from build123d import *

# Parameters (mm, degrees)
F0_W      = 90
F0_H      = 55
F1_DEPTH  = 40
F2_R      = 25
F3_DEPTH  = 45
F4_R      = 25
F5_DEPTH  = 5
F6_W      = 60
F6_H      = 40
F7_DEPTH  = 20
F8_W      = 30
F8_H      = 30
F9_DEPTH  = 10
F10_W     = 15
F10_H     = 30
F11_DEPTH = 30
F13_DEPTH = 45.001
F14_R     = 15
F15_DEPTH = 10
F16_R     = 15
F17_DEPTH = 10
F18_R     = 15
F19_DEPTH = 10
F20_R     = 15
F21_DEPTH = 10


with BuildPart() as f1:
    # F0 (on Front) → F1 (new body)
    with BuildSketch(Plane.XZ):
        Rectangle(F0_W, F0_H)
    extrude(amount=F1_DEPTH)

    # F2 (on face) → F3 (join)
    with BuildSketch(Plane.XZ.offset(40)):
        with Locations((-45, -27.5)):
            Circle(F2_R)
        with Locations((45, -27.5)):
            Circle(F2_R)
    extrude(amount=-F3_DEPTH)

    # F4 (on face) → F5 (join)
    with BuildSketch(Plane.XZ.offset(40)):
        with Locations((-45, -27.5)):
            Circle(F4_R)
        with Locations((45, -27.5)):
            Circle(F4_R)
    extrude(amount=F5_DEPTH)

    # F6 (on face) → F7 (cut)
    with BuildSketch(Plane.XY.offset(27.5)):
        with Locations((15, -20)):
            Rectangle(F6_W, F6_H)
    extrude(amount=-F7_DEPTH, mode=Mode.SUBTRACT)

    # F8 (on face) → F9 (cut)
    with BuildSketch(Plane.XY.offset(7.5)):
        with Locations((0, -20)):
            Rectangle(F8_W, F8_H)
    extrude(amount=-F9_DEPTH, mode=Mode.SUBTRACT)

    # F10 (on face) → F11 (cut)
    with BuildSketch(Plane.XY.offset(27.5)):
        with Locations((-22.5, -20)):
            Rectangle(F10_W, F10_H)
    extrude(amount=-F11_DEPTH, mode=Mode.SUBTRACT)

    # F12 (on face) → F13 (cut, through all)
    with BuildSketch(Plane.XZ.offset(40)):
        Polygon((-15, 27.5), (-30, 27.5), (-15, 12.5), align=None)
        Polygon((-45, 22.5), (-40, 27.5), (-45, 27.5), align=None)
    extrude(amount=-F13_DEPTH, mode=Mode.SUBTRACT)

    # F14 (on face) → F15 (cut)
    with BuildSketch(Plane.XZ.offset(45)):
        with Locations((-45, -27.5)):
            Circle(F14_R)
    extrude(amount=-F15_DEPTH, mode=Mode.SUBTRACT)

    # F16 (on face) → F17 (cut)
    with BuildSketch(Plane.XZ.offset(45)):
        with Locations((45, -27.5)):
            Circle(F16_R)
    extrude(amount=-F17_DEPTH, mode=Mode.SUBTRACT)

    # F18 (on face) → F19 (cut)
    with BuildSketch(Plane(origin=(0, 5, 0), x_dir=(-1, 0, 0), z_dir=(0, 1, 0))):
        with Locations((-45, -27.5)):
            Circle(F18_R)
    extrude(amount=-F19_DEPTH, mode=Mode.SUBTRACT)

    # F20 (on face) → F21 (cut)
    with BuildSketch(Plane(origin=(0, 5, 0), x_dir=(-1, 0, 0), z_dir=(0, 1, 0))):
        with Locations((45, -27.5)):
            Circle(F20_R)
    extrude(amount=-F21_DEPTH, mode=Mode.SUBTRACT)


solid = f1.part
Design review of the part built by this model. Coordinates are the model's own, in mm. A direction names the side the tool comes from. Round coordinates to 2 decimals unless told otherwise and drop trailing zeros. Loops run counter-clockwise (first coordinate to the right, second up) from the corner with the lowest first, then second, coordinate; pieces in that order, holes last. Notation, with made-up numbers: (11, 67) - (49, 67) arc R11 ccw to (49, 81) - close; hole circle Ø1 at (-24.5, 11). An arc over 180 degrees is marked (long way). One line per question, with ' | ' between items.
1. For faces 5 (the face through (-1, 0, 0)), 6 (the face through (45, -35, -27)), 7 (the face through (-15, -38, 10)), 8 (the face through (59.985, 0.07, -26.84)), 9 (the face through (15, -20, 3)), list the 3-axis set-ups (+Z, -Z, +X, -X, +Y, -Y) from which the entire face can be reached by the end or side of a thin tool; tool diameter is ignored.
Results are:
face 5: +Z, +Y | face 6: -Y | face 7: +Z, +X, +Y, -Y | face 8: +Y | face 9: +Z
2. We need section D-D, the plane x = -25.5. State the section outline as (y, z) points, and give its area (3 significant figures).
Results are:
outline: (-45, -43.14) - (5, -43.14) - (5, -11.86) - (0, -11.86) - (0, 23) - (-5, 23) - (-5, -2.5) - (-35, -2.5) - (-35, 23) - (-40, 23) - (-40, -11.86) - (-45, -11.86) - close | area: 2,190 mm²
3. We need section B-B, the plane y = -16. State the section outline as (x, z) points.
Results are:
outline: (-45, -2.5) arc R25 ccw (long way) to (-20, -27.5) - (20, -27.5) arc R25 ccw (long way) to (45, -2.5) - (45, 7.5) - (15, 7.5) - (15, -2.5) - (-30, -2.5) - (-30, 27.5) - (-40, 27.5) - (-45, 22.5) - close
4. We need section C-C, the plane z = 9.5. State the section outline as (x, y) points, and give its area (3 significant figures).
Results are:
outline: (-45, -40) - (-15, -40) - (-15, -35) - (-30, -35) - (-30, -5) - (-15, -5) - (-15, 0) - (-45, 0) - close | area: 750 mm²
5. Clearance check with flat-ended pins moving along their axes: P1, Ø4.5, axis at x = -24, z = 12, coming from the -Y side; P2, Ø12, axis at y = -27.5, z = -19.5, coming from the -X side; P3, Ø24, axis at y = -24.5, z = 10, coming from the +X side. State where each tip first meets the part, or that it passes through.
Results are:
P1: stops at y = -40 | P2: stops at x = -69.92 | P3: stops at x = 45
6. We need section A-A, the plane z = -29.5. State the section outline as (x, y) points, and give its area (3 significant figures).
Results are:
outline: (-69.92, -45) - (-59.87, -45) - (-59.87, -35) - (-30.13, -35) - (-30.13, -45) - (-20.08, -45) - (-20.08, 5) - (-30.13, 5) - (-30.13, -5) - (-59.87, -5) - (-59.87, 5) - (-69.92, 5) - close; (20.08, -45) - (30.13, -45) - (30.13, -35) - (59.87, -35) - (59.87, -45) - (69.92, -45) - (69.92, 5) - (59.87, 5) - (59.87, -5) - (30.13, -5) - (30.13, 5) - (20.08, 5) - close | area: 3,790 mm²
7. Draft analysis for pull direction Y (two halves, no side actions). For faces 1 (the face through (-45, -35, -27)), 2 (the face through (-30, -20, 13)), 3 (the face through (-45, -20, 10)), 4 (the face through (45, -5, -27)), state which applies: released by +Y, released by -Y, zero draft, split by the parting line, or undercut.
Results are:
face 1: released by -Y | face 2: undercut | face 3: zero draft | face 4: released by +Y
8. For L1, parallel to X at y = -43, z = -27 (3 decimals); L2, parallel to X at y = 3, z = -14.5; L3, parallel to Z at x = -45, y = 0.5, list the stretches that pass through material, from the lowest coordinate up. Write a range as [from, to].
Results are:
L1: x = [-69.995, -59.992], [-30.008, -20.005], [20.005, 30.008], [59.992, 69.995] | L2: x = [-66.35, -52.48], [-37.52, -23.65], [23.65, 37.52], [52.48, 66.35] | L3: z = [-52.5, -42.5], [-12.5, -2.5]
